```python
from build123d import *

# Parameters (mm, degrees)
SKETCH_1_R           = 47
EXTRUDE_1_DEPTH      = 5
FILLET_1_R           = 60
SKETCH_31_R          = 1.5
CUT_EXTRUDE_14_DEPTH = 5
SKETCH_35_R          = 2.5
SKETCH_35_R_2        = 2
CUT_EXTRUDE_17_DEPTH = 10
CUT_EXTRUDE_18_DEPTH = 10
FILLET_2_R           = 3
FILLET_3_R           = 20
CUT_EXTRUDE_19_DEPTH = 10
SKETCH_39_R          = 1.5
CUT_EXTRUDE_20_DEPTH = 10
FILLET_4_R           = 3


with BuildPart() as part:
    # 草图1 → 凸台-拉伸1 (new body)
    with BuildSketch(Plane.XY):
        with BuildLine():
            Line((347.693212678, 20), (52.306787322, 20))
            ThreePointArc((52.306787322, 20), (-56, 0), (52.306787322, -20))
            Line((52.306787322, -20), (347.693212678, -20))
            ThreePointArc((347.693212678, -20), (456, 0), (347.693212678, 20))
        make_face()
        Circle(SKETCH_1_R, mode=Mode.SUBTRACT)
        with Locations((400, 0)):
            Circle(SKETCH_1_R, mode=Mode.SUBTRACT)
    extrude(amount=EXTRUDE_1_DEPTH)

    # 圆角1
    fillet_1_edges = [part.edges().sort_by_distance(p)[0] for p in [
        (347.693212678, -20, 2.5),
        (52.306787322, -20, 2.5),
        (52.306787322, 20, 2.5),
        (347.693212678, 20, 2.5),
    ]]
    fillet(fillet_1_edges, radius=FILLET_1_R)

    # 草图31 → 切除-拉伸14 (cut)
    with BuildSketch(Plane.XY.offset(5)):
        with Locations((36.415999231, 36.415999231)):
            Circle(SKETCH_31_R)
        with Locations((36.415999231, -36.415999231)):
            Circle(SKETCH_31_R)
        with Locations((-36.415999231, -36.415999231)):
            Circle(SKETCH_31_R)
        with Locations((-36.415999231, 36.415999231)):
            Circle(SKETCH_31_R)
        with Locations((436.415999231, 36.415999231)):
            Circle(SKETCH_31_R)
        with Locations((436.415999231, -36.415999231)):
            Circle(SKETCH_31_R)
        with Locations((363.584000769, -36.415999231)):
            Circle(SKETCH_31_R)
        with Locations((363.584000769, 36.415999231)):
            Circle(SKETCH_31_R)
    extrude(amount=-CUT_EXTRUDE_14_DEPTH, mode=Mode.SUBTRACT)

    # 草图35 → 切除-拉伸17 (cut)
    with BuildSketch(Plane.XY.offset(5)):
        with Locations((145, 12)):
            Circle(SKETCH_35_R)
        with Locations((255, 12)):
            Circle(SKETCH_35_R)
        with Locations((145, -12)):
            Circle(SKETCH_35_R)
        with Locations((255, -12)):
            Circle(SKETCH_35_R)
        with Locations((90, -12)):
            Circle(SKETCH_35_R_2)
        with Locations((90, 12)):
            Circle(SKETCH_35_R_2)
        with Locations((310, -12)):
            Circle(SKETCH_35_R_2)
        with Locations((310, 12)):
            Circle(SKETCH_35_R_2)
    extrude(amount=-CUT_EXTRUDE_17_DEPTH, mode=Mode.SUBTRACT)

    # 草图37 → 切除-拉伸18 (cut)
    with BuildSketch(Plane(origin=(0, 0, 0), x_dir=(-1, 0, 0), z_dir=(0, 0, -1))):
        Polygon((-232.879996879, 15), (-200, 2.67000117), (-167.120003121, 15), align=None)
        Polygon((-160, 12.32999883), (-192.879996879, 0), (-160, -12.32999883), align=None)
        Polygon((-167.120003121, -15), (-200, -2.67000117), (-232.879996879, -15), align=None)
        Polygon((-240, 12.32999883), (-240, -12.32999883), (-207.120003121, 0), align=None)
    extrude(amount=-CUT_EXTRUDE_18_DEPTH, mode=Mode.SUBTRACT)

    # 圆角2
    fillet_2_edges = [part.edges().sort_by_distance(p)[0] for p in [
        (167.120003121, -15, 2.5),
        (232.879996879, -15, 2.5),
        (192.879996879, 0, 2.5),
        (160, 12.32999883, 2.5),
        (160, -12.32999883, 2.5),
        (240, 12.32999883, 2.5),
        (207.120003121, 0, 2.5),
        (240, -12.32999883, 2.5),
        (232.879996879, 15, 2.5),
        (167.120003121, 15, 2.5),
    ]]
    fillet(fillet_2_edges, radius=FILLET_2_R)

    # 圆角3
    fillet_3_edges = [part.edges().sort_by_distance(p)[0] for p in [
        (200, -2.67000117, 2.5),
        (200, 2.67000117, 2.5),
    ]]
    fillet(fillet_3_edges, radius=FILLET_3_R)

    # 草图38 → 切除-拉伸19 (cut)
    with BuildSketch(Plane(origin=(0, 0, 0), x_dir=(-1, 0, 0), z_dir=(0, 0, -1))):
        Polygon((-302.5, 12.5), (-302.5, -12.5), (-285.833333333, 0), align=None)
        Polygon((-262.5, 12.5), (-279.166666667, 0), (-262.5, -12.5), align=None)
        Polygon((-265.833333333, -15), (-282.5, -2.5), (-299.166666667, -15), align=None)
        Polygon((-299.166666667, 15), (-282.5, 2.5), (-265.833333333, 15), align=None)
        Polygon((-100.833333333, -15), (-117.5, -2.5), (-134.166666667, -15), align=None)
        Polygon((-97.5, 12.5), (-114.166666667, 0), (-97.5, -12.5), align=None)
        Polygon((-117.5, 2.5), (-100.833333333, 15), (-134.166666667, 15), align=None)
        Polygon((-137.5, -12.5), (-120.833333333, 0), (-137.5, 12.5), align=None)
    extrude(amount=-CUT_EXTRUDE_19_DEPTH, mode=Mode.SUBTRACT)

    # 草图39 → 切除-拉伸20 (cut)
    with BuildSketch(Plane.XY.offset(5)):
        with Locations((72.001998462, -12)):
            Circle(SKETCH_39_R)
        with Locations((52, -12)):
            Circle(SKETCH_39_R)
        with Locations((72.001998462, 12)):
            Circle(SKETCH_39_R)
        with Locations((52, 12)):
            Circle(SKETCH_39_R)
        with Locations((348, 12)):
            Circle(SKETCH_39_R)
        with Locations((327.998001538, 12)):
            Circle(SKETCH_39_R)
        with Locations((327.998001538, -12)):
            Circle(SKETCH_39_R)
        with Locations((348, -12)):
            Circle(SKETCH_39_R)
    extrude(amount=-CUT_EXTRUDE_20_DEPTH, mode=Mode.SUBTRACT)

    # 圆角4
    fillet_4_edges = [part.edges().sort_by_distance(p)[0] for p in [
        (100.833333333, -15, 2.5),
        (134.166666667, -15, 2.5),
        (117.5, -2.5, 2.5),
        (299.166666667, 15, 2.5),
        (265.833333333, 15, 2.5),
        (282.5, 2.5, 2.5),
        (279.166666667, 0, 2.5),
        (262.5, 12.5, 2.5),
        (262.5, -12.5, 2.5),
        (282.5, -2.5, 2.5),
        (265.833333333, -15, 2.5),
        (299.166666667, -15, 2.5),
        (137.5, -12.5, 2.5),
        (137.5, 12.5, 2.5),
        (120.833333333, 0, 2.5),
        (97.5, -12.5, 2.5),
        (114.166666667, 0, 2.5),
        (97.5, 12.5, 2.5),
        (117.5, 2.5, 2.5),
        (134.166666667, 15, 2.5),
        (100.833333333, 15, 2.5),
        (302.5, 12.5, 2.5),
        (285.833333333, 0, 2.5),
        (302.5, -12.5, 2.5),
    ]]
    fillet(fillet_4_edges, radius=FILLET_4_R)


solid = part.part
```
The listing builds one solid part. Answer for the finished solid, in the listing's coordinates (mm). A direction names the side the tool comes from. Coordinates: 2 decimals unless noted, no trailing zeros. Write each loop counter-clockwise with the first axis right and the second up, starting at its lowest first coordinate (ties: lowest second). Pieces come first, ordered by that corner, then holes.
Q1. Section B-B, the plane y = 28 is taken. Write down the section's boundary in (x, z).
Returned:
outline: (-48.5, 0) - (-37.75, 0) - (-37.75, 5) - (-48.5, 5) - close; (37.75, 0) - (54.07, 0) - (54.07, 5) - (37.75, 5) - close; (345.93, 0) - (362.25, 0) - (362.25, 5) - (345.93, 5) - close; (437.75, 0) - (448.5, 0) - (448.5, 5) - (437.75, 5) - close
Q2. Which of the six approach directions +Z, -Z, +X, -X, +Y, -Y give full straight-line access (tool end or side, diameter ignored) to faces 1 (the cylindrical face through (60.053, -24.986, 2.535)), 2 (the flat face through (225.129, 6.753, 2.465)), 3 (the cylindrical face through (339.322, 24.718, 2.535))?
Returned:
face 1: +Z, -Z, -Y
face 2: +Z, -Z
face 3: +Z, -Z, +Y
Q3. Section C-C, the plane z = 2.05 is taken. Give the number of separate pieces and of enclosed holes in the cut face, then the cut area to 3 significant figures.
Returned:
separate pieces: 1
enclosed holes: 38
area: 14,800 mm2
Q4. Given P1, Ø2.5, axis at x = 52, y = 12, coming from the -Z side; P2, Ø2.5, axis at x = 283, z = 3, coming from the +Y side; P3, Ø1, axis at x = 156, z = 4, coming from the -Y side, each flat-ended and moving along its own axis, determine where each tip first touches the part or whether it passes through.
Returned:
P1: passes through
P2: stops at y = 20
P3: stops at y = -20
Q5. Find the intervals of material crossed by line 1 along Y through (x, z) = (90, 2.6); line 2 along Y through (x, z) = (118, 1.8); line 3 along X through (y, z) = (30, 0.7), in increasing order.
Returned:
line 1: y = -20 to -14, -10 to 10, 14 to 20
line 2: y = -20 to -15, -3.29 to 3.29, 15 to 20
line 3: x = -47.29 to -36.18, 36.18 to 50.83, 349.17 to 363.82, 436.18 to 447.29
Q6. Section A-A, the plane x = 0 is taken. Write down the section's boundary in (y, z).
Returned:
outline: (-56, 0) - (-47, 0) - (-47, 5) - (-56, 5) - close; (47, 0) - (56, 0) - (56, 5) - (47, 5) - close
Q7. The mould has two halves that part along X. Classify faces 4 (the cylindrical face through (60.678, 24.718, 2.535)), 5 (the flat face through (198.8, -3.9, 0)): released by +X, released by -X, zero draft, split by the parting line, or undercut.
Returned:
face 4: undercut
face 5: zero draft
